from build123d import *

# Parameters (mm, degrees)
SKETCH2_R           = 25
BOSS_EXTRUDE1_DEPTH = 30
SKETCH3_OUTSIDE_W   = 329.93
SKETCH3_OUTSIDE_H   = 343.864
SKETCH3_OUTSIDE_R   = 45.033320997
CUT_EXTRUDE1_DEPTH  = 60
CUT_EXTRUDE1_DRAFT  = -60
SKETCH4_OUTSIDE_W   = 329.93
SKETCH4_OUTSIDE_H   = 343.864
SKETCH4_OUTSIDE_R   = 45.033320997
CUT_EXTRUDE2_DEPTH  = 60
CUT_EXTRUDE2_DRAFT  = -60
SKETCH5_W           = 27.935883882
SKETCH5_H           = 10
CUT_EXTRUDE4_DEPTH  = 25


with BuildPart() as part:
    # Sketch2 → Boss-Extrude1 (new, symmetric)
    with BuildSketch(Plane(origin=(0, 0, 0), x_dir=(1, 0, 0), z_dir=(0, 1, 0))):
        Polygon((0, 52), (-45.033320997, 26), (-45.033320997, -26), (0, -52), (45.033320997, -26), (45.033320997, 26), align=None)
        with Locations(Location((0, 0, 0), (0, 0, 270))):
            Circle(SKETCH2_R, mode=Mode.SUBTRACT)
    extrude(amount=BOSS_EXTRUDE1_DEPTH, both=True)


with BuildPart() as cut_extrude1_tool:
    # Sketch3 outside → Cut-Extrude1 (with draft: the straight prism first)
    with BuildSketch(Plane(origin=(0, 30, 0), x_dir=(1, 0, 0), z_dir=(0, 1, 0))):
        Rectangle(SKETCH3_OUTSIDE_W, SKETCH3_OUTSIDE_H)
        Circle(SKETCH3_OUTSIDE_R, mode=Mode.SUBTRACT)
    extrude(amount=-CUT_EXTRUDE1_DEPTH)
    # Cut-Extrude1: the draft: its side faces are tilted about the plane it starts from
    cut_extrude1_sides = [cut_extrude1_tool.faces().sort_by_distance(p)[0] for p in [
        (0, 0, 171.932),
        (164.965, 0, 0),
        (0, 0, -171.932),
        (-164.965, 0, 0),
        (-45.033320997, 0, 0),
    ]]
    draft(cut_extrude1_sides, Plane(origin=(0, 30, 0), x_dir=(1, 0, 0), z_dir=(0, 1, 0)), CUT_EXTRUDE1_DRAFT)


with BuildPart() as part_1:
    add(part.part)

    # Cut-Extrude1: cut by cut_extrude1_tool
    add(cut_extrude1_tool.part, mode=Mode.SUBTRACT)


with BuildPart() as cut_extrude2_tool:
    # Sketch4 outside → Cut-Extrude2 (with draft: the straight prism first)
    with BuildSketch(Plane.XZ.offset(30)):
        Rectangle(SKETCH4_OUTSIDE_W, SKETCH4_OUTSIDE_H)
        Circle(SKETCH4_OUTSIDE_R, mode=Mode.SUBTRACT)
    extrude(amount=-CUT_EXTRUDE2_DEPTH)
    # Cut-Extrude2: the draft: its side faces are tilted about the plane it starts from
    cut_extrude2_sides = [cut_extrude2_tool.faces().sort_by_distance(p)[0] for p in [
        (0, 0, -171.932),
        (164.965, 0, 0),
        (0, 0, 171.932),
        (-164.965, 0, 0),
        (-45.033320997, 0, 0),
    ]]
    draft(cut_extrude2_sides, Plane.XZ.offset(30), CUT_EXTRUDE2_DRAFT)


with BuildPart() as part_2:
    add(part_1.part)

    # Cut-Extrude2: cut by cut_extrude2_tool
    add(cut_extrude2_tool.part, mode=Mode.SUBTRACT)

    # Sketch5 → Cut-Extrude4 (cut)
    with BuildSketch(Plane.XZ.offset(30)):
        with Locations((33.722829942, 0)):
            Rectangle(SKETCH5_W, SKETCH5_H)
        Polygon((19.515258923, -43.801419977), (5.547316982, -19.608234858), (14.20757102, -14.608234858), (28.175512961, -38.801419977), align=None)
        Polygon((-28.175512961, -38.801419977), (-14.20757102, -14.608234858), (-5.547316982, -19.608234858), (-19.515258923, -43.801419977), align=None)
        with Locations((-33.722829942, 0)):
            Rectangle(SKETCH5_W, SKETCH5_H)
        Polygon((-19.515258923, 43.801419977), (-5.547316982, 19.608234858), (-14.20757102, 14.608234858), (-28.175512961, 38.801419977), align=None)
        Polygon((28.175512961, 38.801419977), (14.20757102, 14.608234858), (5.547316982, 19.608234858), (19.515258923, 43.801419977), align=None)
    extrude(amount=-CUT_EXTRUDE4_DEPTH, mode=Mode.SUBTRACT)


solid = part_2.part
Verification items for the finished model (mm, model axes). A direction names the side the tool comes from. Round coordinates to 2 decimals unless told otherwise and drop trailing zeros. Loops run counter-clockwise (first coordinate to the right, second up) from the corner with the lowest first, then second, coordinate; pieces in that order, holes last. Notation, with made-up numbers: (-11.5, -24) - (10.5, -24) arc R19 ccw to (10.5, 9) - close; hole circle Ø4 at (-6, 84.5). An arc over 180 degrees is marked (long way). Use a Markdown table: item, result. Add a question column.
1. Access from +Z, -Z, +X, -X, +Y, -Y to the whole of each face (thin tool, end or side, straight path). Record for faces 5 (the face through (-22.201, 0.499, -39.182)), 6 (the face through (-35, -18, 5)), 7 (the face through (18, -5, 30)).
2. Thickness scan on probe 1 along Z at (x, y) = (0, 16.5); probe 2 along X at (y, z) = (-19.5, -31.5); probe 3 along X at (y, z) = (14, 0). Record the ranges inside material, lowest first. Write a range as [from, to].
3. Section check A-A, the plane y = -24. Give the number of separate pieces and of enclosed holes in the cut face, plus the area to 3 significant figures.
4. Section check B-B, the plane y = 3. Record the boundary of the cut face in (x, z).
5. Gauge pin test, flat ends, axial feed: pin 1 (10.5 mm diameter, centred on x = -37, y = -18.5, fed in from +Z); pin 2 (5.5 mm diameter, centred on x = -14, z = 27, fed in from -Y); pin 3 (16.5 mm diameter, centred on x = 37, y = -17.5, fed in from -Z); pin 4 (1.5 mm diameter, centred on y = -15.5, z = 4, fed in from +X). Record the tip position at first contact, or that the pin passes through.
6. Release check for a two-part mould opening along X. For faces 1 (the face through (-40.8, -28.9, -23.2)), 2 (the face through (40.38, 29.04, 23.45)), 3 (the face through (7.509, -0.42, 23.846)), 4 (the face through (-17, -5, 30)) record: released by +X, released by -X, zero draft, split by the parting line, or undercut.
Checks:
| question | item | result |
|---|---|---|
| 1 | face 5 | -Z, -X, +Y, -Y |
| 1 | face 6 | +X, -X, -Y |
| 1 | face 7 | -Y |
| 2 | probe 1 | z = [-52, -25], [25, 52] |
| 2 | probe 2 | x = [-35.51, -23.96], [-12.41, 12.41], [23.96, 35.51] |
| 2 | probe 3 | x = [-45.03, -25], [25, 45.03] |
| 3 | separate pieces | 6 |
| 3 | enclosed holes | 0 |
| 3 | area | 3,850 mm^2 |
| 4 | outline | (-45.03, -26) - (0, -52) - (45.03, -26) - (45.03, 26) - (0, 52) - (-45.03, 26) - close; hole circle Ø50 at (0, 0) |
| 5 | pin 1 | stops at z = 33.67 |
| 5 | pin 2 | stops at y = -5 |
| 5 | pin 3 | stops at z = -35.4 |
| 5 | pin 4 | passes through |
| 6 | face 1 | released by -X |
| 6 | face 2 | released by +X |
| 6 | face 3 | undercut |
| 6 | face 4 | undercut |
